Geometry: final body of the model. Coordinates: model frame, mm. Coordinates: 2 decimals unless noted, no trailing zeros. Write each loop counter-clockwise with the first axis right and the second up, starting at its lowest first coordinate (ties: lowest second). Pieces come first, ordered by that corner, then holes. Notation, with made-up numbers: (-8.75, 26) -> (50.25, 26) arc R27 ccw to (50.25, 53) -> close; hole circle Ø8 at (-28, 50). An arc over 180 degrees is marked (long way). One line per item, written item: value. Start each with the question number.
from build123d import *

# Parameters (mm, degrees)
CYLINDER002_R     = 4
CYLINDER002_DEPTH = 30
CYLINDER001_R     = 6
CYLINDER001_DEPTH = 30
CYLINDER_R        = 10
CYLINDER_DEPTH    = 30
CHAMFER_SIZE      = 1
CHAMFER001_SIZE   = 1


with BuildPart() as cilindro002:
    # Cylinder002 → Cylinder002 (new body)
    with BuildSketch(Plane(origin=(0, 15, 21), x_dir=(1, 0, 0), z_dir=(0, -1, 0))):
        Circle(CYLINDER002_R)
    extrude(amount=CYLINDER002_DEPTH)


with BuildPart() as cilindro001:
    # Cylinder001 → Cylinder001 (new body)
    with BuildSketch(Plane.XY):
        Circle(CYLINDER001_R)
    extrude(amount=CYLINDER001_DEPTH)


with BuildPart() as chamfer001:
    # Cylinder → Cylinder (new body)
    with BuildSketch(Plane.XY):
        Circle(CYLINDER_R)
    extrude(amount=CYLINDER_DEPTH)

    # Cut: cut Cilindro001
    add(cilindro001.part, mode=Mode.SUBTRACT)

    # Cut001: cut Cilindro002
    add(cilindro002.part, mode=Mode.SUBTRACT)

    # Chamfer
    chamfer_edges = [chamfer001.edges().sort_by_distance(p)[0] for p in [
        (-10, 0, 30),
    ]]
    chamfer(chamfer_edges, length=CHAMFER_SIZE)

    # Chamfer001
    chamfer001_edges = [chamfer001.edges().sort_by_distance(p)[0] for p in [
        (-10, 0, 0),
    ]]
    chamfer(chamfer001_edges, length=CHAMFER001_SIZE)


solid = chamfer001.part
Q1. Cut plane D-D on z = 26. Output: boundary loops of the cut face in (x, y), and give its area (3 significant figures).
Q2. Cut plane C-C on z = 21. Output: boundary loops of the cut face in (x, y).
Q3. Cut plane B-B on y = 0. Output: boundary loops of the cut face in (x, z).
Q4. Draft query along X for faces 1 (the cylindrical face through (9.54, 3, 14.8)), 2 (the cylindrical face through (3.815, 7.277, 22.201)), 3 (the flat face through (2, -6, 0)). Return one class per face: pulls with the +X half, pulls with the -X half, needs draft (parallel to the pull), parting line crosses it, or undercut.
Q5. Line query: L1, parallel to Z at x = 0, y = -7.9; L2, parallel to Y at x = 0, z = 14; L3, parallel to X at y = 6.5, z = 21. Output: solid intervals per line, ascending. Write a range as from..to.
Q6. Cut plane A-A on x = 0. Output: boundary loops of the cut face in (y, z).
Q7. First-contact query: P1, Ø4, axis at y = -7, z = 6, coming from the -X side; P2, Ø9.5, axis at x = 0, y = 0, coming from the +Z side; P3, Ø6, axis at x = 4, y = 7.5, coming from the -Z side; P4, Ø10, axis at y = 6, z = 13.5, coming from the -X side. Flat tips, straight axial feed; report the tip coordinate or a pass-through.
Solution:
1. outline: circle Ø20 at (0, 0); hole circle Ø12 at (0, 0)
1. area: 201 mm²
2. outline: (-4, -9.17) -> (-4, -4.47) arc R6 cw to (-4, 4.47) -> (-4, 9.17) arc R10 ccw to start; (4, -9.17) arc R10 ccw to (4, 9.17) -> (4, 4.47) arc R6 cw to (4, -4.47) -> close
3. outline: (-10, 1) -> (-9, 0) -> (-6, 0) -> (-6, 30) -> (-9, 30) -> (-10, 29) -> close; (6, 0) -> (9, 0) -> (10, 1) -> (10, 29) -> (9, 30) -> (6, 30) -> close
4. face 1: parting line crosses it
4. face 2: undercut
4. face 3: needs draft
5. L1: 0..17, 25..30
5. L2: -10..-6, 6..10
5. L3: -7.6..-4, 4..7.6
6. outline: (-10, 1) -> (-9, 0) -> (-6, 0) -> (-6, 17) -> (-10, 17) -> close; (-10, 25) -> (-6, 25) -> (-6, 30) -> (-9, 30) -> (-10, 29) -> close; (6, 0) -> (9, 0) -> (10, 1) -> (10, 17) -> (6, 17) -> close; (6, 25) -> (10, 25) -> (10, 29) -> (9, 30) -> (6, 30) -> close
7. P1: x = -8.66
7. P2: through
7. P3: z = 0
7. P4: x = -9.95
